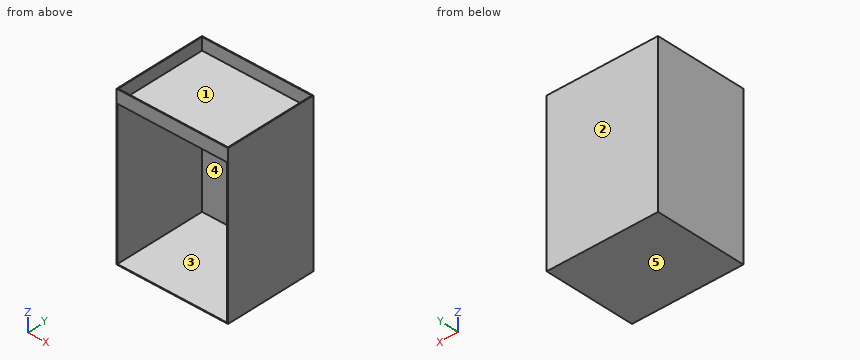
```python
from build123d import *

# Parameters (mm, degrees)
F0_W     = 431.8
F0_H     = 609.6
F1_DEPTH = 355.6
F2_W     = 425.45
F2_H     = 555.625
F3_DEPTH = 352.425
F4_W     = 425.45
F4_H     = 349.25
F5_DEPTH = 47.625


with BuildPart() as f1:
    # F0 (on Front) → F1 (new body)
    with BuildSketch(Plane.XZ):
        Rectangle(F0_W, F0_H)
    extrude(amount=F1_DEPTH)

    # F2 (on face) → F3 (cut)
    with BuildSketch(Plane.XZ.offset(355.6)):
        with Locations((0, -23.8125)):
            Rectangle(F2_W, F2_H)
    extrude(amount=-F3_DEPTH, mode=Mode.SUBTRACT)

    # F4 (on face) → F5 (cut)
    with BuildSketch(Plane.XY.offset(304.8)):
        with Locations((0, -177.8)):
            Rectangle(F4_W, F4_H)
    extrude(amount=-F5_DEPTH, mode=Mode.SUBTRACT)


solid = f1.part
```
Model file for the job. Use its own axes, mm. Face numbers are marked on the shaded views. A direction names the side the tool comes from. Round coordinates to 2 decimals unless told otherwise and drop trailing zeros. Write each loop counter-clockwise with the first axis right and the second up, starting at its lowest first coordinate (ties: lowest second). Pieces come first, ordered by that corner, then holes. Notation, with made-up numbers: (-11.5, 70.5) - (-5.5, 70.5) arc R12 cw to (-5.5, 83.5) - close; hole circle Ø5 at (88, 72). An arc over 180 degrees is marked (long way). One line per item, written item: value.
(1) Cut at B-B, the plane y = -283. Give the cut face in (x, z) (3 decimals), plus the area to 3 significant figures.
Values follow:
outline: (-215.9, -304.8) - (215.9, -304.8) - (215.9, 304.8) - (212.725, 304.8) - (212.725, 257.175) - (-212.725, 257.175) - (-212.725, 304.8) - (-215.9, 304.8) - close; hole (-212.725, -301.625) - (212.725, -301.625) - (212.725, 254) - (-212.725, 254) - close
area: 6,570 mm²
(2) Cut at A-A, the plane x = 69. Give the cut face in (y, z) (3 decimals).
Values follow:
outline: (-355.6, -304.8) - (0, -304.8) - (0, 304.8) - (-3.175, 304.8) - (-3.175, 257.175) - (-352.425, 257.175) - (-352.425, 304.8) - (-355.6, 304.8) - (-355.6, 254) - (-3.175, 254) - (-3.175, -301.625) - (-355.6, -301.625) - close
(3) Cut at C-C, the plane z = 54. Give the cut face in (x, y) (3 decimals).
Values follow:
outline: (-215.9, -355.6) - (-212.725, -355.6) - (-212.725, -3.175) - (212.725, -3.175) - (212.725, -355.6) - (215.9, -355.6) - (215.9, 0) - (-215.9, 0) - close
(4) Wall check: probe 1 along Z at (x, y) = (193.5, -52) (3 decimals); probe 2 along X at (y, z) = (-109.5, 236) (3 decimals); probe 3 along Y at (x, z) = (-36.5, 112) (3 decimals). Give the ranges that are in metal, low to high.
Values follow:
probe 1: z = -304.8 to -301.625, 254 to 257.175
probe 2: x = -215.9 to -212.725, 212.725 to 215.9
probe 3: y = -3.175 to 0
(5) Drop a flat-ended pin along its axis: P1, Ø1.5, axis at x = -61.5, y = -131, coming from the +Z side (3 decimals). Give the stop position or say it passes through.
Values follow:
P1: stops at z = 257.175
(6) Two-plate mould, pull along Z, no slides. Class the marked faces 1, 2 and 3: pulls with the +Z half, pulls with the -Z half, needs draft (parallel to the pull), parting line crosses it, or undercut.
Values follow:
face 1: pulls with the +Z half
face 2: needs draft
face 3: undercut
(7) 3-axis set-ups, long thin cutter, end or side, ignore diameter. For the marked faces 4 and 5: which of +Z, -Z, +X, -X, +Y, -Y reach the whole face in a straight line?
Values follow:
face 4: -Y
face 5: -Z, +X, -X, +Y, -Y
